Autodesk Inventor part; units mm, degrees
ref_plane "YZ Plane" through (0, 0, 0) normal (1, 0, 0) x (0, 1, 0)
ref_plane "XZ Plane" through (0, 0, 0) normal (0, 1, 0) x (-1, 0, 0)
ref_plane "XY Plane" through (0, 0, 0) normal (0, 0, 1) x (1, 0, 0)
sketch "Sketch1" plane through (0, 0, 0) normal (0, 1, 0) x (-1, 0, 0)
  line L0 (-4.1, 2.85) -> (-3.1, 2.85)
  line L1 (-3.1, 2.85) -> (-3.1, 2.35)
  line L2 (-3.1, 2.35) -> (2.5, 2.35)
  line L3 (2.5, 2.35) -> (2.5, -2.35)
  line L4 (-4.1, 2.85) -> (-3.6981, 4.35)
  line L5 (-3.6981, 4.35) -> (-7.6981, 4.35)
  line L6 (-7.6981, 4.35) -> (-7.6981, 2.35)
  line L7 (-7.6981, 2.35) -> (-18.6981, 2.35)
  line L8 (-18.6981, 2.35) -> (-19.6981, 1.35)
  line L9 (-19.6981, 1.35) -> (-19.6981, -0.65)
  line L10 (-19.6981, -0.65) -> (-17.966, -1.65)
  line L11 (-17.966, -1.65) -> (-7.6981, -1.65)
  line L12 (-7.6981, -1.65) -> (-7.6981, -3.25)
  line L13 (-7.6981, -3.25) -> (-3.9124, -3.25)
  line L14 (-3.9124, -3.25) -> (-4.1, -2.55)
  line L15 (-4.1, -2.55) -> (-3.6, -2.55)
  line L16 (-3.6, -2.55) -> (-3.6, -2.35)
  line L17 (-3.6, -2.35) -> (2.5, -2.35)
  circle A0 centre (0, 0) radius 1.4
  dimension "d1" = 4
  dimension "d2" = 2
  dimension "d3" = 75
  dimension "d4" = 4.7
  dimension "d5" = 5.6
  dimension "d6" = 1
  dimension "d7" = 0.5
  dimension "d8" = 75
  dimension "d9" = 7.6
  dimension "d10" = 2
  dimension "d11" = 0.5
  dimension "d12" = 0.2
  dimension "d13" = 2.8
  dimension "d14" = 2.5
  dimension "d15" = 2.35
  dimension "d17" = 0
  dimension "d18" = 0
  dimension "d19" = 4
  dimension "d20" = 0
  dimension "d21" = 0
  dimension "d23" = 2
  dimension "d24" = 60
  dimension "d25" = 45
  dimension "d26" = 12
  dimension "d27" = 1
extrude "Plate1" add sketch "Sketch1" along normal blind 1
chamfer "Corner Chamfer1" distance 1 angle 45 2 edges at (-2.5, 0.5, 2.35) (-2.5, 0.5, -2.35)
sketch "Sketch2" plane through (0, 1, 0) normal (0, 1, 0) x (1, 0, 0)
  circle A0 centre (0, 0) radius 1.4
equation "\"d8\" = d3"
equation "\"d15\" = 0.5 * d4"
equation "\"d31\" = Thickness"
equation "\"BendRadius\" = Thickness"
equation "\"BendReliefWidth\" = Thickness"
equation "\"BendReliefDepth\" = 0.5 * Thickness"
equation "\"CornerReliefSize\" = 4 * Thickness"
equation "\"MinimumRemnant\" = 2 * Thickness"
equation "\"TransitionRadius\" = BendRadius"
equation "\"JacobiRadiusSize\" = BendRadius"
equation "\"GapSize\" = Thickness"
equation "\"d16\" = BendRadius"
properties part number "PlacaFasePlug" material "Steel, Galvanized"
CAD build for the part. Positions are in the model's coordinates, mm. A direction names the side the tool comes from. Round coordinates to 2 decimals unless told otherwise and drop trailing zeros. Loops run counter-clockwise (first coordinate to the right, second up) from the corner with the lowest first, then second, coordinate; pieces in that order, holes last. Notation, with made-up numbers: (-8, 82) - (26, 82) arc R32 ccw to (26, 110) - close; hole circle Ø4 at (47, 6.5). An arc over 180 degrees is marked (long way). Return JSON: item names as keys, results as strings. Group by question number.
Q1. Flat gauge pins, fed straight in: pin 1 Ø0.5 at (x, y) = (12, 0.5) entering from -Z; pin 2 Ø4 at (x, z) = (14.5, -2.5) entering from -Y; pin 3 Ø0.5 at (y, z) = (0.5, -2.5) entering from +X; pin 4 Ø0.5 at (x, y) = (14, 0.5) entering from +Z. Where does each tip first touch, or does it go through?
Q2. Band-saw the part on D-D on x = 9.75. Give the cut face in (y, z).
Q3. Drill centre lines: line 1 along Z through (x, y) = (0, 0.6); line 2 along Z through (x, y) = (8.75, 0.75); line 3 along X through (y, z) = (0.1, 0.5). Where is each one in solid material? Low to high. Write a range as [from, to].
Q4. Two-plate mould, pull along Z, no slides. Class faces 1 (the face through (3.9, 0.5, 3.6)), 2 (the face through (9, 0, 1)), 3 (the face through (1.1, 0.5, -2.35)): +Z half, -Z half, draft (parallel to the pull), parting line (faces both ways), or undercut.
Q5. Band-saw the part on A-A on x = 0. Give the cut face in (y, z), plus the area to 3 significant figures.
Q6. Band-saw the part on B-B on y = 0.85. Give the cut face in (x, z).
Q7. Tool access for faces 4 (the face through (0.8, 0.5, 2.35)), 5 (the face through (7.698, 0.5, -2.4)), 6 (the face through (3.6, 0.5, 2.85)), 7 (the face through (7.698, 0.5, 3.4)): list every direction of +Z, -Z, +X, -X, +Y, -Y with a clear straight run to the whole face (end or side of a thin tool).
Q8. Band-saw the part on C-C on z = 0. Give the cut face in (x, y).
Solutions:
{
 "1": {"pin 1": "stops at z = -1.65", "pin 2": "stops at y = 0", "pin 3": "stops at x = 7.7", "pin 4": "stops at z = 2.35"},
 "2": {"outline": "(0, -1.65) - (1, -1.65) - (1, 2.35) - (0, 2.35) - close"},
 "3": {"line 1": "z = [-2.35, -1.4], [1.4, 2.35]", "line 2": "z = [-1.65, 2.35]", "line 3": "x = [-2.5, -1.31], [1.31, 19.7]"},
 "4": {"face 1": "undercut", "face 2": "draft", "face 3": "-Z half"},
 "5": {"outline": "(0, -2.35) - (1, -2.35) - (1, -1.4) - (0, -1.4) - close; (0, 1.4) - (1, 1.4) - (1, 2.35) - (0, 2.35) - close", "area": "1.90 mm^2"},
 "6": {"outline": "(-2.5, -1.35) - (-1.5, -2.35) - (3.6, -2.35) - (3.6, -2.55) - (4.1, -2.55) - (3.91, -3.25) - (7.7, -3.25) - (7.7, -1.65) - (17.97, -1.65) - (19.7, -0.65) - (19.7, 1.35) - (18.7, 2.35) - (7.7, 2.35) - (7.7, 4.35) - (3.7, 4.35) - (4.1, 2.85) - (3.1, 2.85) - (3.1, 2.35) - (-1.5, 2.35) - (-2.5, 1.35) - close; hole circle Ø2.8 at (0, 0)"},
 "7": {"face 4": "+Z, -X, +Y, -Y", "face 5": "-Z, +X, +Y, -Y", "face 6": "-X, +Y, -Y", "face 7": "+Z, +X, +Y, -Y"},
 "8": {"outline": "(-2.5, 0) - (-1.4, 0) - (-1.4, 1) - (-2.5, 1) - close; (1.4, 0) - (19.7, 0) - (19.7, 1) - (1.4, 1) - close"}
}
